from build123d import *

# Parameters (mm, degrees)
F3_DEPTH = 6
F4_R     = 2


with BuildPart() as f1:
    # F0 (on Front) → F1 (revolve)
    with BuildSketch(Plane.XZ):
        with BuildLine():
            Line((0, 1.375929), (0, 5))
            Line((0, 5), (-28, 5))
            ThreePointArc((-28, 5), (-29.414214, 5.585786), (-30, 7))
            Line((-30, 7), (-30, 98))
            ThreePointArc((-30, 98), (-30.585786, 99.414214), (-32, 100))
            Line((-32, 100), (-33, 100))
            ThreePointArc((-33, 100), (-34.414214, 99.414214), (-35, 98))
            Line((-35, 98), (-35, 0))
            Line((-35, 0), (-32.452703, 0))
            Line((-32.452703, 0), (-31.345069, 1.375929))
            Line((-31.345069, 1.375929), (0, 1.375929))
        make_face()
    revolve(axis=Axis((0, 0, 64.654013), (0, 0, -1)))

    # F2 (on Front) → F3 (join, symmetric)
    with BuildSketch(Plane.XZ):
        with BuildLine():
            Line((-43.091623, 60), (-33.091623, 60))
            Line((-33.091623, 60), (-33.091623, 67))
            Line((-33.091623, 67), (-43.091623, 67))
            ThreePointArc((-43.091623, 67), (-55.112439, 62.020815), (-60.091623, 50))
            Line((-60.091623, 50), (-60.091623, 30))
            ThreePointArc((-60.091623, 30), (-55.112439, 17.979185), (-43.091623, 13))
            Line((-43.091623, 13), (-33.091623, 13))
            Line((-33.091623, 13), (-33.091623, 20))
            Line((-33.091623, 20), (-43.091623, 20))
            ThreePointArc((-43.091623, 20), (-50.162691, 22.928932), (-53.091623, 30))
            Line((-53.091623, 30), (-53.091623, 50))
            ThreePointArc((-53.091623, 50), (-50.162691, 57.071068), (-43.091623, 60))
        make_face()
    extrude(amount=F3_DEPTH, both=True)

    # F4
    f4_edges = [f1.edges().sort_by_distance(p)[0] for p in [
        (-38.786751, -6, 67),
        (-53.091623, -6, 40),
        (-55.112439, 6, 62.020815),
        (-53.091623, 6, 40),
    ]]
    fillet(f4_edges, radius=F4_R)


solid = f1.part
Geometry check sheet. Reference: the model listing, model coordinates, mm. A direction names the side the tool comes from. Give positions to 0.01 mm unless a question says otherwise; leave off trailing zeros. Order: outer loops, then holes, each group sorted by start corner. A loop starts at its lowest first (then second) coordinate and runs counter-clockwise, first axis right, second up. Notation, with made-up numbers: (2, 58.25) - (28, 58.25) arc R21 cw to (28, 95.25) - close; hole circle Ø6 at (70.25, -35.5). An arc over 180 degrees is marked (long way). Answer as a JSON object with one key per item and string values.
(1) Cross-section at D-D (z = 76). Record the cut outline in (x, y).
Report:
{"outline": "circle Ø70 at (0, 0); hole circle Ø60 at (0, 0)"}
(2) Tool access check on faces 4 (the flat face through (-56, -6, 40)), 5 (the cylindrical face through (-50.24, -0.056, 56.993)), 6 (the flat face through (0, 0, 5)), 7 (the flat face through (0, 0, 1.376)). Record the directions out of +Z, -Z, +X, -X, +Y, -Y that give a thin tool (end or side, any length) a straight path to the whole face; none if there is none.
Report:
{"face 4": "+Z, -Z, -X, -Y", "face 5": "+Y, -Y", "face 6": "+Z", "face 7": "-Z"}
(3) Depth check by flat-ended pin: pin 1 Ø12 at (y, z) = (-25, 79.5) entering from -X; pin 2 Ø2.5 at (x, y) = (-41, 0.5) entering from +Z; pin 3 Ø3 at (y, z) = (15, 58.5) entering from -X; pin 4 Ø9 at (x, y) = (-38, 1) entering from -Z. Enter the tip coordinate at first touch or a pass-through.
Report:
{"pin 1": "x = -29.39", "pin 2": "z = 67", "pin 3": "x = -32.29", "pin 4": "z = 0"}
(4) Cross-section at C-C (x = 0). Record the cut outline in (y, z), then the cut area to 3 significant figures.
Report:
{"outline": "(-35, 0) - (-32.45, 0) - (-31.35, 1.38) - (31.35, 1.38) - (32.45, 0) - (35, 0) - (35, 98) arc R2 ccw to (33, 100) - (32, 100) arc R2 ccw to (30, 98) - (30, 7) arc R2 cw to (28, 5) - (-28, 5) arc R2 cw to (-30, 7) - (-30, 98) arc R2 ccw to (-32, 100) - (-33, 100) arc R2 ccw to (-35, 98) - close", "area": "1,210 mm^2"}
(5) Draft check along Z on faces 1 (the cylindrical face through (29.97, 1.32, 53.14)), 2 (the flat face through (-23.2, -23.2, 0)), 3 (the flat face through (-39, 0, 60)). Enter one of: released by +Z, released by -Z, zero draft, split by the parting line, or undercut.
Report:
{"face 1": "zero draft", "face 2": "released by -Z", "face 3": "undercut"}
(6) Material ranges on line 1 (Y direction, x = 0, z = 76); line 2 (Z direction, x = 7.5, y = -26); line 3 (X direction, y = -4.5, z = 85), recorded low to high.
Report:
{"line 1": "-35 to -30, 30 to 35", "line 2": "1.38 to 5", "line 3": "-34.71 to -29.66, 29.66 to 34.71"}
(7) Cross-section at A-A (z = 44). Record the cut outline in (x, y), then the cut area to 3 significant figures.
Report:
{"outline": "(-60.09, -4) arc R2 ccw to (-58.09, -6) - (-55.09, -6) arc R2 ccw to (-53.09, -4) - (-53.09, 4) arc R2 ccw to (-55.09, 6) - (-58.09, 6) arc R2 ccw to (-60.09, 4) - close; circle Ø70 at (0, 0); hole circle Ø60 at (0, 0)", "area": "1,100 mm^2"}
